Check sheet for the modelled part. Datum: model origin and axes. Units: mm. A direction names the side the tool comes from. Coordinates: 2 decimals unless noted, no trailing zeros. Loops run counter-clockwise (first coordinate to the right, second up) from the corner with the lowest first, then second, coordinate; pieces in that order, holes last. Notation, with made-up numbers: (50.5, -3) - (62.5, -3) arc R23 cw to (62.5, 14) - close; hole circle Ø5 at (-36.75, 13). An arc over 180 degrees is marked (long way). Write each question's results on one line, items separated by ' | '. Start each with the question number.
1. Cross-section at A-A (z = -1.55). Record the cut outline in (x, y).
2. Cross-section at C-C (y = 10). Record the cut outline in (x, z), and give its area (3 significant figures).
3. Thickness scan on line 1 (X direction, y = 9.5, z = 0.35); line 2 (Y direction, x = 12.5, z = 0.1); line 3 (X direction, y = 4.5, z = 1.2). Record the ranges inside material, lowest first. Write a range as [from, to].
4. Cross-section at D-D (y = 4.5). Record the cut outline in (x, z), and give its area (3 significant figures).
5. Draft check along X on faces 1 (the face through (13, 12.5, 0)), 2 (the face through (4, 10, -2)), 3 (the face through (7.1, 18, 0)), 4 (the face through (-4.5, 10, 0)). Enter one of: released by +X, released by -X, zero draft, split by the parting line, or undercut.
6. Tool access check on faces 5 (the face through (12, 4.85, 0)), 6 (the face through (-2, 4.85, 0)), 7 (the face through (-2, 15.15, 0)), 8 (the face through (15.1, 10, 0)). Record the directions out of +Z, -Z, +X, -X, +Y, -Y that give a thin tool (end or side, any length) a straight path to the whole face; none if there is none.
7. Gauge pin test, flat ends, axial feed: P1, Ø1.2, axis at x = 11.5, z = -0.5, coming from the -Y side; P2, Ø1.2, axis at x = 12.5, z = 0.5, coming from the +Y side; P3, Ø1.2, axis at y = 17.5, z = 0.5, coming from the -X side. Record the tip position at first contact, or that the pin passes through.
8. Cross-section at B-B (x = 11.5). Record the cut outline in (y, z).
```python
from build123d import *

# Parameters (mm, degrees)
SKETCH_1_W      = 4
SKETCH_1_H      = 5
EXTRUDE_1_DEPTH = 2


with BuildPart() as part:
    # 草图1 → 凸台-拉伸1 (new, symmetric)
    with BuildSketch(Plane.XY):
        Polygon((0, 15.15), (0, 20), (7.1, 20), (7.1, 15.15), (12.1, 15.15), (17, 15.15), (17, 4.85), (12.1, 4.85), (7.1, 4.85), (7.1, 0), (0, 0), (0, 4.85), (-4.5, 4.85), (-4.5, 15.15), align=None)
        with Locations((13.1, 10)):
            Rectangle(SKETCH_1_W, SKETCH_1_H, mode=Mode.SUBTRACT)
    extrude(amount=EXTRUDE_1_DEPTH, both=True)


solid = part.part
```
Established:
1) outline: (-4.5, 4.85) - (0, 4.85) - (0, 0) - (7.1, 0) - (7.1, 4.85) - (17, 4.85) - (17, 15.15) - (7.1, 15.15) - (7.1, 20) - (0, 20) - (0, 15.15) - (-4.5, 15.15) - close; hole (11.1, 7.5) - (15.1, 7.5) - (15.1, 12.5) - (11.1, 12.5) - close
2) outline: (-4.5, -2) - (11.1, -2) - (11.1, 2) - (-4.5, 2) - close; (15.1, -2) - (17, -2) - (17, 2) - (15.1, 2) - close | area: 70.0 mm^2
3) line 1: [-4.5, 11.1], [15.1, 17] | line 2: [4.85, 7.5], [12.5, 15.15] | line 3: [0, 7.1]
4) outline: (0, -2) - (7.1, -2) - (7.1, 2) - (0, 2) - close | area: 28.4 mm^2
5) face 1: undercut | face 2: zero draft | face 3: released by +X | face 4: released by -X
6) face 5: +Z, -Z, +X, -Y | face 6: +Z, -Z, -X, -Y | face 7: +Z, -Z, -X, +Y | face 8: +Z, -Z
7) P1: y = 4.85 | P2: y = 15.15 | P3: x = 0
8) outline: (4.85, -2) - (7.5, -2) - (7.5, 2) - (4.85, 2) - close; (12.5, -2) - (15.15, -2) - (15.15, 2) - (12.5, 2) - close
